Geometry check sheet. Reference: the model listing, model coordinates, mm. Round coordinates to 2 decimals unless told otherwise and drop trailing zeros. Answer as CSV lines item,"result". Start each with the question number.
1) Draft check along X on faces 1 (the cylindrical face through (-28, 29, 30)), 2 (the flat face through (0, 30, 30)), 3 (the cylindrical face through (-26.11, -26.01, 29.58)), 4 (the cylindrical face through (28, -29, 30)). Enter one of: released by +X, released by -X, zero draft, split by the parting line, or undercut.
2) Thickness scan on line 1 along Y through (x, z) = (25, 15); line 2 along X through (y, z) = (-27, 24.5). Record the ranges inside material, lowest first.
3) Depth check by flat-ended pin: P1, Ø2.5, axis at x = -25, y = -25, coming from the +Z side. Enter the tip coordinate at first touch or a pass-through.
Autodesk Inventor part; units mm, degrees
ref_plane "YZ Plane" through (0, 0, 0) normal (1, 0, 0) x (0, 1, 0)
ref_plane "XZ Plane" through (0, 0, 0) normal (0, 1, 0) x (-1, 0, 0)
ref_plane "XY Plane" through (0, 0, 0) normal (0, 0, 1) x (1, 0, 0)
sketch "Sketch1" plane through (0, 0, 0) normal (0, 0, 1) x (1, 0, 0)
  line L0 (-30, -30) -> (30, -30)
  line L1 (30, -30) -> (30, 30)
  line L2 (30, 30) -> (-30, 30)
  line L3 (-30, 30) -> (-30, -30)
  line L4 (-30, -30) -> (30, 30) construction
  line L5 (30, -30) -> (-30, 30) construction
  line L6 (30, 30) -> (25, 30) construction
  line L7 (25, 30) -> (25, 25) construction
  line L8 (-30, 30) -> (-25, 30) construction
  line L9 (-25, 30) -> (-25, 25) construction
  line L10 (-30, -30) -> (-30, -25) construction
  line L11 (-30, -25) -> (-25, -25) construction
  line L12 (30, -30) -> (30, -25) construction
  line L13 (30, -25) -> (25, -25) construction
  circle A0 centre (-25, 25) radius 1.5
  circle A1 centre (25, 25) radius 1.5
  circle A2 centre (25, -25) radius 1.5
  circle A3 centre (-25, -25) radius 1.5
  point P0 (0, 0)
  dimension "d0" = 60
  dimension "d1" = 60
  dimension "d2" = 5
  dimension "d3" = 5
  dimension "d4" = 5
  dimension "d5" = 5
  dimension "d6" = 5
  dimension "d7" = 5
  dimension "d8" = 5
  dimension "d9" = 5
  dimension "d10" = 3
  dimension "d11" = 3
  dimension "d12" = 3
  dimension "d13" = 3
extrude "Block" add sketch "Sketch1" along normal blind 60
fillet "Fillets FTW" radius 5 4 edges at (-30, 30, 30) (-30, -30, 30) (30, -30, 30) (30, 30, 30)
properties part number "60x60Spacer"
Answer block:
1,face 1,"released by -X"
1,face 2,"zero draft"
1,face 3,"undercut"
1,face 4,"released by +X"
2,line 1,"y = -30 to -26.5, -23.5 to 23.5, 26.5 to 30"
2,line 2,"x = -29.58 to 29.58"
3,P1,"passes through"
